Geometry: final body of the model. Coordinates: model frame, mm. A direction names the side the tool comes from. Coordinates: 2 decimals unless noted, no trailing zeros. Loops run counter-clockwise (first coordinate to the right, second up) from the corner with the lowest first, then second, coordinate; pieces in that order, holes last. Notation, with made-up numbers: (-28.75, 80) - (26.25, 80) arc R35 ccw to (26.25, 119) - close; hole circle Ø11 at (60.25, 74.5). An arc over 180 degrees is marked (long way). Return JSON: item names as keys, results as strings.
from build123d import *

# Parameters (mm, degrees)
SKETCH2_W           = 52.5
SKETCH2_H           = 10
SKETCH2_W_2         = 10
SKETCH2_H_2         = 30
SKETCH2_H_3         = 12.5
SKETCH2_W_3         = 12.5
BOSS_EXTRUDE1_DEPTH = 5
SKETCH2_4_W         = 10
SKETCH2_4_H         = 5
SKETCH2_4_W_2       = 5
SKETCH2_4_H_2       = 10
BOSS_EXTRUDE2_DEPTH = 52
SKETCH2_5_W         = 10
SKETCH2_5_H         = 10
BOSS_EXTRUDE3_DEPTH = 52
SKETCH2_6_W         = 10
SKETCH2_6_H         = 10
CUT_EXTRUDE1_DEPTH  = 42
SKETCH3_R           = 2
CUT_EXTRUDE2_DEPTH  = 10


with BuildPart() as part:
    # Sketch2 → Boss-Extrude1 (new body)
    with BuildSketch(Plane(origin=(0, 0, 0), x_dir=(1, 0, 0), z_dir=(0, 1, 0))):
        with Locations((-31.25, 20)):
            Rectangle(SKETCH2_W, SKETCH2_H)
        with Locations((-62.5, 20)):
            Rectangle(SKETCH2_W_2, SKETCH2_H)
        with Locations((-62.5, 0)):
            Rectangle(SKETCH2_W_2, SKETCH2_H_2)
        Rectangle(SKETCH2_W_2, SKETCH2_H_2)
        with Locations((0, 20)):
            Rectangle(SKETCH2_W_2, SKETCH2_H)
        with Locations((-31.25, -20)):
            Rectangle(SKETCH2_W, SKETCH2_H)
        with Locations((0, -20)):
            Rectangle(SKETCH2_W_2, SKETCH2_H)
        with Locations((-62.5, -20)):
            Rectangle(SKETCH2_W_2, SKETCH2_H)
        with Locations((31.25, -20)):
            Rectangle(SKETCH2_W, SKETCH2_H)
        with Locations((31.25, 20)):
            Rectangle(SKETCH2_W, SKETCH2_H)
        with Locations((62.5, 0)):
            Rectangle(SKETCH2_W_2, SKETCH2_H_2)
        with Locations((62.5, 20)):
            Rectangle(SKETCH2_W_2, SKETCH2_H)
        with Locations((62.5, -20)):
            Rectangle(SKETCH2_W_2, SKETCH2_H)
        with Locations((0, -31.25)):
            Rectangle(SKETCH2_W_2, SKETCH2_H_3)
        with Locations((62.5, -31.25)):
            Rectangle(SKETCH2_W_2, SKETCH2_H_3)
        with Locations((73.75, -20)):
            Rectangle(SKETCH2_W_3, SKETCH2_H)
        with Locations((73.75, 20)):
            Rectangle(SKETCH2_W_3, SKETCH2_H)
        with Locations((0, 31.25)):
            Rectangle(SKETCH2_W_2, SKETCH2_H_3)
        with Locations((62.5, 31.25)):
            Rectangle(SKETCH2_W_2, SKETCH2_H_3)
        with Locations((-62.5, 31.25)):
            Rectangle(SKETCH2_W_2, SKETCH2_H_3)
        with Locations((-73.75, 20)):
            Rectangle(SKETCH2_W_3, SKETCH2_H)
        with Locations((-73.75, -20)):
            Rectangle(SKETCH2_W_3, SKETCH2_H)
        with Locations((-62.5, -31.25)):
            Rectangle(SKETCH2_W_2, SKETCH2_H_3)
    extrude(amount=BOSS_EXTRUDE1_DEPTH)

    # Sketch2<4> → Boss-Extrude2 (add)
    with BuildSketch(Plane(origin=(0, 0, 0), x_dir=(1, 0, 0), z_dir=(0, 1, 0))):
        with Locations((-62.5, -40)):
            Rectangle(SKETCH2_4_W, SKETCH2_4_H)
        with Locations((0, -40)):
            Rectangle(SKETCH2_4_W, SKETCH2_4_H)
        with Locations((62.5, -40)):
            Rectangle(SKETCH2_4_W, SKETCH2_4_H)
        with Locations((82.5, -20)):
            Rectangle(SKETCH2_4_W_2, SKETCH2_4_H_2)
        with Locations((82.5, 20)):
            Rectangle(SKETCH2_4_W_2, SKETCH2_4_H_2)
        with Locations((62.5, 40)):
            Rectangle(SKETCH2_4_W, SKETCH2_4_H)
        with Locations((0, 40)):
            Rectangle(SKETCH2_4_W, SKETCH2_4_H)
        with Locations((-62.5, 40)):
            Rectangle(SKETCH2_4_W, SKETCH2_4_H)
        with Locations((-82.5, 20)):
            Rectangle(SKETCH2_4_W_2, SKETCH2_4_H_2)
        with Locations((-82.5, -20)):
            Rectangle(SKETCH2_4_W_2, SKETCH2_4_H_2)
    extrude(amount=BOSS_EXTRUDE2_DEPTH)

    # Sketch2<5> → Boss-Extrude3 (add)
    with BuildSketch(Plane(origin=(0, 0, 0), x_dir=(1, 0, 0), z_dir=(0, 1, 0))):
        with Locations((-62.5, -47.5)):
            Rectangle(SKETCH2_5_W, SKETCH2_5_H)
        with Locations((-90, -20)):
            Rectangle(SKETCH2_5_W, SKETCH2_5_H)
        with Locations((-90, 20)):
            Rectangle(SKETCH2_5_W, SKETCH2_5_H)
        with Locations((-62.5, 47.5)):
            Rectangle(SKETCH2_5_W, SKETCH2_5_H)
        with Locations((0, 47.5)):
            Rectangle(SKETCH2_5_W, SKETCH2_5_H)
        with Locations((62.5, 47.5)):
            Rectangle(SKETCH2_5_W, SKETCH2_5_H)
        with Locations((90, 20)):
            Rectangle(SKETCH2_5_W, SKETCH2_5_H)
        with Locations((90, -20)):
            Rectangle(SKETCH2_5_W, SKETCH2_5_H)
        with Locations((62.5, -47.5)):
            Rectangle(SKETCH2_5_W, SKETCH2_5_H)
        with Locations((0, -47.5)):
            Rectangle(SKETCH2_5_W, SKETCH2_5_H)
    extrude(amount=BOSS_EXTRUDE3_DEPTH)

    # Sketch2<6> → Cut-Extrude1 (cut)
    with BuildSketch(Plane(origin=(0, 0, 0), x_dir=(1, 0, 0), z_dir=(0, 1, 0))):
        with Locations((-62.5, -47.5)):
            Rectangle(SKETCH2_6_W, SKETCH2_6_H)
        with Locations((-90, -20)):
            Rectangle(SKETCH2_6_W, SKETCH2_6_H)
        with Locations((-90, 20)):
            Rectangle(SKETCH2_6_W, SKETCH2_6_H)
        with Locations((-62.5, 47.5)):
            Rectangle(SKETCH2_6_W, SKETCH2_6_H)
        with Locations((0, 47.5)):
            Rectangle(SKETCH2_6_W, SKETCH2_6_H)
        with Locations((62.5, 47.5)):
            Rectangle(SKETCH2_6_W, SKETCH2_6_H)
        with Locations((90, 20)):
            Rectangle(SKETCH2_6_W, SKETCH2_6_H)
        with Locations((90, -20)):
            Rectangle(SKETCH2_6_W, SKETCH2_6_H)
        with Locations((62.5, -47.5)):
            Rectangle(SKETCH2_6_W, SKETCH2_6_H)
        with Locations((0, -47.5)):
            Rectangle(SKETCH2_6_W, SKETCH2_6_H)
    extrude(amount=CUT_EXTRUDE1_DEPTH, mode=Mode.SUBTRACT)

    # Sketch3 → Cut-Extrude2 (cut)
    with BuildSketch(Plane.XZ.offset(-42)):
        with Locations(Location((-62.5, -47.5, 0), (0, 0, 270))):
            Circle(SKETCH3_R)
        with Locations(Location((-90, -20, 0), (0, 0, 270))):
            Circle(SKETCH3_R)
        with Locations(Location((0, -47.5, 0), (0, 0, 270))):
            Circle(SKETCH3_R)
        with Locations(Location((62.5, -47.5, 0), (0, 0, 270))):
            Circle(SKETCH3_R)
        with Locations(Location((90, -20, 0), (0, 0, 270))):
            Circle(SKETCH3_R)
        with Locations(Location((90, 20, 0), (0, 0, 270))):
            Circle(SKETCH3_R)
        with Locations(Location((62.5, 47.5, 0), (0, 0, 270))):
            Circle(SKETCH3_R)
        with Locations(Location((0, 47.5, 0), (0, 0, 270))):
            Circle(SKETCH3_R)
        with Locations(Location((-90, 20, 0), (0, 0, 270))):
            Circle(SKETCH3_R)
        with Locations(Location((-62.5, 47.5, 0), (0, 0, 270))):
            Circle(SKETCH3_R)
    extrude(amount=-CUT_EXTRUDE2_DEPTH, mode=Mode.SUBTRACT)


solid = part.part
Item 1: Section query C-C, the plane z = -47.5. Return loops of the section in (x, y).
Worked out:
{"outline": "(-67.5, 42) - (-64.5, 42) - (-64.5, 52) - (-67.5, 52) - close; (-60.5, 42) - (-57.5, 42) - (-57.5, 52) - (-60.5, 52) - close; (-5, 42) - (-2, 42) - (-2, 52) - (-5, 52) - close; (2, 42) - (5, 42) - (5, 52) - (2, 52) - close; (57.5, 42) - (60.5, 42) - (60.5, 52) - (57.5, 52) - close; (64.5, 42) - (67.5, 42) - (67.5, 52) - (64.5, 52) - close"}
Item 2: Mould query, pull axis X, two halves, no side actions, for faces 4 (the face through (87.7, 42, -20.1)), 5 (the face through (-80, 28, -20)), 6 (the face through (85, 21, -20)). Classes: +X half, -X half, draft (parallel to the pull), parting line (faces both ways), or undercut.
Worked out:
{"face 4": "draft", "face 5": "undercut", "face 6": "+X half"}
Item 3: First-contact query: pin 1 Ø22 at (y, z) = (38, -35.5) entering from -X; pin 2 Ø1.5 at (x, y) = (-64.5, 39) entering from +Z; pin 3 Ø5 at (x, z) = (-90, 20) entering from -Y. Flat tips, straight axial feed; report the tip coordinate or a pass-through.
Worked out:
{"pin 1": "x = -85", "pin 2": "z = 42.5", "pin 3": "y = 42"}
Item 4: Section query D-D, the plane x = 62.5. Return loops of the section in (y, z).
Worked out:
{"outline": "(0, -42.5) - (42, -42.5) - (42, -45.5) - (52, -45.5) - (52, -37.5) - (5, -37.5) - (5, 37.5) - (52, 37.5) - (52, 45.5) - (42, 45.5) - (42, 42.5) - (0, 42.5) - close; (42, -52.5) - (52, -52.5) - (52, -49.5) - (42, -49.5) - close; (42, 49.5) - (52, 49.5) - (52, 52.5) - (42, 52.5) - close"}
Item 5: Section query A-A, the plane z = 31. Return loops of the section in (x, y).
Worked out:
{"outline": "(-67.5, 0) - (-57.5, 0) - (-57.5, 5) - (-67.5, 5) - close; (-5, 0) - (5, 0) - (5, 5) - (-5, 5) - close; (57.5, 0) - (67.5, 0) - (67.5, 5) - (57.5, 5) - close"}
Item 6: Ray query, probe 1 along X at (y, z) = (45.25, 20); probe 2 along X at (y, z) = (46.5, -47.5); probe 3 along Z at (x, y) = (-61.5, 29). Return the intervals inside material, ascending. Write a range as from..to.
Worked out:
{"probe 1": "-95..-92, -88..-80, 80..88, 92..95", "probe 2": "-67.5..-64.5, -60.5..-57.5, -5..-2, 2..5, 57.5..60.5, 64.5..67.5", "probe 3": "-42.5..-37.5, 37.5..42.5"}
Item 7: Reachability of faces 1 (the face through (-5, 28, 40)), 2 (the face through (60, 42, 47)), 3 (the face through (-85, 21, 20)) from +Z, -Z, +X, -X, +Y, -Y: full face, straight path, thin tool, end or side. Return the list, or none.
Worked out:
{"face 1": "+Z, +Y, -Y", "face 2": "+Z, +X, -X, -Y", "face 3": "+Z, -Z, -X, -Y"}
Item 8: Section query B-B, the plane x = 83. Return loops of the section in (y, z), and give its area (3 significant figures).
Worked out:
{"outline": "(0, -25) - (52, -25) - (52, -15) - (0, -15) - close; (0, 15) - (52, 15) - (52, 25) - (0, 25) - close", "area": "1,040 mm^2"}
